Can you work these out from the model? Positions are in its coordinate system, mm. Face numbers are marked on the shaded views. A direction names the side the tool comes from. Round coordinates to 2 decimals unless told otherwise and drop trailing zeros. Loops run counter-clockwise (first coordinate to the right, second up) from the corner with the lowest first, then second, coordinate; pieces in that order, holes last.
(1) Which directions (+Z, -Z, +X, -X, +Y, -Y) give clear straight access to the entire face, cutting with the end or side of a thin tool? Please do the marked faces 5 and 6.
(2) If I drill on line 1 along X through (y, z) = (3.7, -222.75); line 2 along Y through (x, z) = (-282, -218.5); line 3 along Z through (x, y) = (-279.5, 2.35), over which ranges is the centre line in solid material (lowest first)?
(3) I want a section at D-D on z = -228.5. Write out the boundary of the cut face in (x, y), plus the area to 3 significant figures.
(4) I want a section at C-C on y = 2. Write out the boundary of the cut face in (x, z).
(5) I want a section at A-A on z = -218.5. Write out the boundary of the cut face in (x, y).
(6) Thinking about a two-plate mould opening in Z: for the marked faces 1, 2, 3 and 4, which applies, released by +Z, released by -Z, zero draft, split by the parting line, or undercut?
(7) I want a section at B-B on x = -277.5. Write out the boundary of the cut face in (y, z).
(8) Will these pins go through, and if not, where does the flat tip stop? pin 1 Ø10 at (x, z) = (-275.5, -227) entering from -Y; pin 2 Ø1 at (x, y) = (-269, 5) entering from +Z; pin 3 Ø3.5 at (y, z) = (1, -224) entering from +X; pin 4 Ø2.5 at (y, z) = (1.5, -220.5) entering from -X.
from build123d import *

# Parameters (mm, degrees)
SKETCH1_R           = 5
BOSS_EXTRUDE1_DEPTH = 3
SKETCH2_R           = 10
SKETCH2_R_2         = 5
BOSS_EXTRUDE2_DEPTH = 3


with BuildPart() as part:
    # Sketch1 → Boss-Extrude1 (new body)
    with BuildSketch(Plane(origin=(0, 0, 0), x_dir=(1, 0, 0), z_dir=(0, 1, 0))):
        with BuildLine():
            Line((-281.53939526, 229.203780512), (-281.53939526, 216.403780512))
            ThreePointArc((-281.53939526, 216.403780512), (-276.03939526, 214.375557893), (-270.53939526, 216.403780512))
            Line((-270.53939526, 216.403780512), (-270.53939526, 229.203780512))
            ThreePointArc((-270.53939526, 229.203780512), (-276.03939526, 231.252855213), (-281.53939526, 229.203780512))
        make_face()
        with Locations((-276.03939526, 222.846937384)):
            Circle(SKETCH1_R, mode=Mode.SUBTRACT)
    extrude(amount=BOSS_EXTRUDE1_DEPTH)

    # Sketch2 → Boss-Extrude2 (add)
    with BuildSketch(Plane(origin=(0, 3, 0), x_dir=(1, 0, 0), z_dir=(0, 1, 0))):
        with Locations((-276.03939526, 222.846937384)):
            Circle(SKETCH2_R)
        with Locations((-276.03939526, 222.846937384)):
            Circle(SKETCH2_R_2, mode=Mode.SUBTRACT)
    extrude(amount=BOSS_EXTRUDE2_DEPTH)


solid = part.part
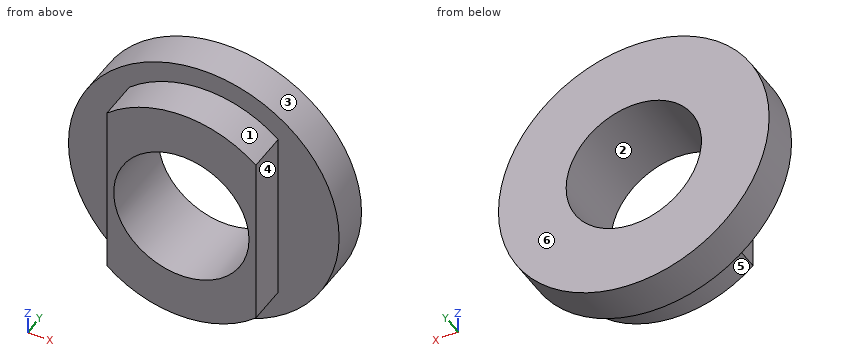
Filled sheet:
1. face 5: -Z, -Y
1. face 6: +Z, -Z, +X, -X, +Y
2. line 1: x = -286.04 to -281.04, -271.04 to -266.04
2. line 2: y = 3 to 6
2. line 3: z = -230.51 to -226.46, -219.24 to -215.11
3. outline: (-284.29, 3) - (-281.54, 3) - (-281.54, 0) - (-270.54, 0) - (-270.54, 3) - (-267.79, 3) - (-267.79, 6) - (-284.29, 6) - close
3. area: 82.5 mm2
4. outline: (-281.54, -229.2) arc R8.41 ccw to (-270.54, -229.2) - (-270.54, -216.4) arc R8.47 ccw to (-281.54, -216.4) - close; hole circle Ø10 at (-276.04, -222.85)
5. outline: (-285.05, 3) - (-281.54, 3) - (-281.54, 0) - (-278.51, 0) - (-278.51, 6) - (-285.05, 6) - close; (-273.57, 0) - (-270.54, 0) - (-270.54, 3) - (-267.03, 3) - (-267.03, 6) - (-273.57, 6) - close
6. face 1: released by +Z
6. face 2: undercut
6. face 3: split by the parting line
6. face 4: zero draft
7. outline: (0, -231.12) - (3, -231.12) - (3, -232.74) - (6, -232.74) - (6, -227.63) - (0, -227.63) - close; (0, -218.07) - (6, -218.07) - (6, -212.95) - (3, -212.95) - (3, -214.5) - (0, -214.5) - close
8. pin 1: stops at y = 0
8. pin 2: stops at z = -215.28
8. pin 3: stops at x = -270.54
8. pin 4: stops at x = -281.54
